CAD build for the part. Positions are in the model's coordinates, mm. Face numbers are marked on the shaded views. A direction names the side the tool comes from. Coordinates: 2 decimals unless noted, no trailing zeros. Loops run counter-clockwise (first coordinate to the right, second up) from the corner with the lowest first, then second, coordinate; pieces in that order, holes last. Notation, with made-up numbers: (-11, 87) -> (28, 87) arc R13 ccw to (28, 108) -> close; hole circle Ø9 at (-17, 41). An arc over 180 degrees is marked (long way). Write each question's results on one line, items separated by ' | '.
```python
from build123d import *

# Parameters (mm, degrees)
BOSS_EXTRUDE1_DEPTH  = 4.7625
M4_CLEARANCE_HOLE1_D = 4.8
SKETCH5_R            = 1.085
CUT_EXTRUDE1_DEPTH   = 45.811860093


with BuildPart() as part:
    # Sketch1 → Boss-Extrude1 (new body)
    with BuildSketch(Plane.XY):
        with BuildLine():
            Line((-20.319587173, -31.597761766), (-19.064971157, -30.343145751))
            ThreePointArc((-19.064971157, -30.343145751), (-16.469584367, -28.60896374), (-13.408116908, -28))
            Line((-13.408116908, -28), (13.408116908, -28))
            ThreePointArc((13.408116908, -28), (16.469584367, -28.60896374), (19.064971157, -30.343145751))
            Line((19.064971157, -30.343145751), (20.319587173, -31.597761766))
            ThreePointArc((20.319587173, -31.597761766), (28.097761766, -31.597761766), (28.097761766, -23.819587173))
            Line((28.097761766, -23.819587173), (26.843145751, -22.564971157))
            ThreePointArc((26.843145751, -22.564971157), (25.10896374, -19.969584367), (24.5, -16.908116908))
            Line((24.5, -16.908116908), (24.5, 16.908116908))
            ThreePointArc((24.5, 16.908116908), (25.10896374, 19.969584367), (26.843145751, 22.564971157))
            Line((26.843145751, 22.564971157), (28.097761766, 23.819587173))
            ThreePointArc((28.097761766, 23.819587173), (28.097761766, 31.597761766), (20.319587173, 31.597761766))
            Line((20.319587173, 31.597761766), (19.064971157, 30.343145751))
            ThreePointArc((19.064971157, 30.343145751), (16.469584367, 28.60896374), (13.408116908, 28))
            Line((13.408116908, 28), (-13.408116908, 28))
            ThreePointArc((-13.408116908, 28), (-16.469584367, 28.60896374), (-19.064971157, 30.343145751))
            Line((-19.064971157, 30.343145751), (-20.319587173, 31.597761766))
            ThreePointArc((-20.319587173, 31.597761766), (-28.097761766, 31.597761766), (-28.097761766, 23.819587173))
            Line((-28.097761766, 23.819587173), (-26.843145751, 22.564971157))
            ThreePointArc((-26.843145751, 22.564971157), (-25.10896374, 19.969584367), (-24.5, 16.908116908))
            Line((-24.5, 16.908116908), (-24.5, -16.908116908))
            ThreePointArc((-24.5, -16.908116908), (-25.10896374, -19.969584367), (-26.843145751, -22.564971157))
            Line((-26.843145751, -22.564971157), (-28.097761766, -23.819587173))
            ThreePointArc((-28.097761766, -23.819587173), (-28.097761766, -31.597761766), (-20.319587173, -31.597761766))
        make_face()
    extrude(amount=BOSS_EXTRUDE1_DEPTH)

    # M4 Clearance Hole1 (through all)
    with Locations(Plane.XY.offset(4.7625)):
        with Locations((-24.20867447, 27.70867447), (24.20867447, 27.70867447), (24.20867447, -27.70867447), (-24.20867447, -27.70867447)):
            Hole(M4_CLEARANCE_HOLE1_D / 2)

    # Sketch5 → Cut-Extrude1 (cut, through all)
    with BuildSketch(Plane.XY.offset(4.7625)):
        with BuildLine():
            Line((-13.66148, -4.78318826), (-11.66148, -4.958165587))
            Line((-11.66148, -4.958165587), (-11.66148, -5.5))
            ThreePointArc((-11.66148, -5.5), (-9.699095434, -10.237615434), (-4.96148, -12.2))
            Line((-4.96148, -12.2), (6.23852, -12.2))
            ThreePointArc((6.23852, -12.2), (10.976135434, -10.237615434), (12.93852, -5.5))
            Line((12.93852, -5.5), (12.93852, 5.5))
            ThreePointArc((12.93852, 5.5), (10.976135434, 10.237615434), (6.23852, 12.2))
            Line((6.23852, 12.2), (-4.96148, 12.2))
            ThreePointArc((-4.96148, 12.2), (-9.699095434, 10.237615434), (-11.66148, 5.5))
            Line((-11.66148, 5.5), (-11.66148, 4.958165587))
            Line((-11.66148, 4.958165587), (-13.66148, 4.78318826))
            Line((-13.66148, 4.78318826), (-13.66148, 2.41681174))
            Line((-13.66148, 2.41681174), (-11.66148, 2.241834413))
            Line((-11.66148, 2.241834413), (-11.66148, -2.241834413))
            Line((-11.66148, -2.241834413), (-13.66148, -2.41681174))
            Line((-13.66148, -2.41681174), (-13.66148, -4.78318826))
        make_face()
        with Locations((-10.16148, -13.7)):
            Circle(SKETCH5_R)
        with Locations((-10.16148, 13.7)):
            Circle(SKETCH5_R)
        with Locations((7.93852, 15.2)):
            Circle(SKETCH5_R)
        with Locations((7.93852, -15.2)):
            Circle(SKETCH5_R)
    extrude(amount=-CUT_EXTRUDE1_DEPTH, mode=Mode.SUBTRACT)


solid = part.part
```
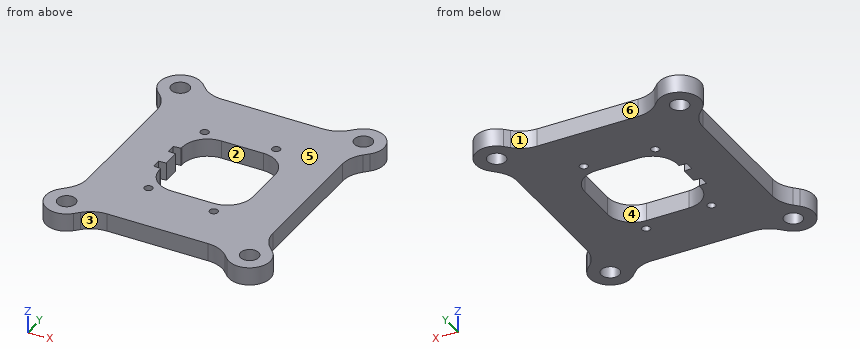
Q1. Cut at B-B on z = 1.75. Give the number of separate pieces and of enclosed holes in the cut face, and give its area (3 significant figures).
Results are:
separate pieces: 1 | enclosed holes: 9 | area: 2,390 mm^2
Q2. Cut at A-A on x = -6. Write the cut outline in (y, z).
Results are:
outline: (-28, 0) -> (-12.12, 0) -> (-12.12, 4.76) -> (-28, 4.76) -> close; (12.12, 0) -> (28, 0) -> (28, 4.76) -> (12.12, 4.76) -> close
Q3. Wall check: L1, parallel to X at y = 14.5, z = 2.2; L2, parallel to X at y = -0.5, z = 0.6; L3, parallel to Y at x = 25.5, z = 4. Give the ranges that are in metal, low to high. Write a range as from..to.
Results are:
L1: -24.5..-10.89, -9.43..7.11, 8.77..24.5 | L2: -24.5..-11.66, 12.94..24.5 | L3: -33.05..-29.73, -25.69..-20.78, 20.78..25.69, 29.73..33.05
Q4. Which spindle directions (+Z, -Z, +X, -X, +Y, -Y) get a long thin tool onto all of the face, cutting with end or side? Do the marked faces 1, 2 and 3. Say none if no direction does.
Results are:
face 1: +Z, -Z, +Y | face 2: +Z, -Z | face 3: +Z, -Z, -Y
Q5. Pull direction Y, two halves, no side cores. Call the marked faces 4, 5 and 6: +Y half, -Y half, draft (parallel to the pull), parting line (faces both ways), or undercut.
Results are:
face 4: undercut | face 5: draft | face 6: +Y half
Q6. Drop flat-ended pins along their axis: pin 1 (1.9 mm diameter, centred on y = -4, z = 2, fed in from +X); pin 2 (1.3 mm diameter, centred on x = -10.16, y = 13.7, fed in from +Z); pin 3 (2.5 mm diameter, centred on x = 3, z = 1.5, fed in from +Y); pin 4 (2.5 mm diameter, centred on y = 2.5, z = 3, fed in from -X). Give the stop position or say it passes through.
Results are:
pin 1: x = 24.5 | pin 2: through | pin 3: y = 28 | pin 4: x = -24.5
